```python
from build123d import *

# Parameters (mm, degrees)
BOSS_EXTRUDE1_DEPTH                              = 22.098
BOSS_EXTRUDE2_DEPTH                              = 5.08
FILLET1_R                                        = 2.54
CBORE_FOR_M4_HEX_HEAD_MACHINE_SCREW1_D           = 4.5
CBORE_FOR_M4_HEX_HEAD_MACHINE_SCREW1_CBORE_D     = 10.59
CBORE_FOR_M4_HEX_HEAD_MACHINE_SCREW1_CBORE_DEPTH = 3
M4_CLEARANCE_HOLE1_D                             = 4.8


with BuildPart() as part:
    # Sketch1 → Boss-Extrude1 (new body)
    with BuildSketch(Plane(origin=(0, 0, 0), x_dir=(1, 0, 0), z_dir=(0, 1, 0))):
        with BuildLine():
            Line((-6.35, 4.572), (-6.35, 0))
            Line((-6.35, 0), (6.35, 0))
            Line((6.35, 0), (6.35, 4.572))
            ThreePointArc((6.35, 4.572), (0, 10.922), (-6.35, 4.572))
        make_face()
    extrude(amount=BOSS_EXTRUDE1_DEPTH)

    # Sketch2 → Boss-Extrude2 (add)
    with BuildSketch(Plane(origin=(0, 22.098, 0), x_dir=(1, 0, 0), z_dir=(0, 1, 0))):
        with BuildLine():
            Line((-6.35, 0), (-6.35, -19.05))
            Line((-6.35, -19.05), (6.35, -19.05))
            Line((6.35, -19.05), (6.35, 0))
            Line((6.35, 0), (6.35, 4.572))
            ThreePointArc((6.35, 4.572), (0, 10.922), (-6.35, 4.572))
            Line((-6.35, 4.572), (-6.35, 0))
        make_face()
    extrude(amount=BOSS_EXTRUDE2_DEPTH)

    # Fillet1
    fillet1_edges = [part.edges().sort_by_distance(p)[0] for p in [
        (6.35, 24.638, 19.05),
        (-6.35, 24.638, 19.05),
    ]]
    fillet(fillet1_edges, radius=FILLET1_R)

    # CBORE for M4 Hex Head Machine Screw1 (through all)
    with Locations(Plane(origin=(0, 27.178, 0), x_dir=(1, 0, 0), z_dir=(0, 1, 0))):
        with Locations((0, 4.572)):
            CounterBoreHole(CBORE_FOR_M4_HEX_HEAD_MACHINE_SCREW1_D / 2, CBORE_FOR_M4_HEX_HEAD_MACHINE_SCREW1_CBORE_D / 2, CBORE_FOR_M4_HEX_HEAD_MACHINE_SCREW1_CBORE_DEPTH)

    # M4 Clearance Hole1 (through all)
    with Locations(Plane(origin=(0, 24.178, 0), x_dir=(1, 0, 0), z_dir=(0, 1, 0))):
        with Locations((0, 4.572)):
            Hole(M4_CLEARANCE_HOLE1_D / 2)


solid = part.part
```
Geometry check sheet. Reference: the model listing, model coordinates, mm. A direction names the side the tool comes from. Give positions to 0.01 mm unless a question says otherwise; leave off trailing zeros. Write each loop counter-clockwise with the first axis right and the second up, starting at its lowest first coordinate (ties: lowest second). Pieces come first, ordered by that corner, then holes. Notation, with made-up numbers: (-34.5, -37) -> (-10.5, -37) arc R21 cw to (-10.5, -24) -> close; hole circle Ø10 at (24, 71.5). An arc over 180 degrees is marked (long way). Use one line per item in the form item = value.
Item 1: Depth check by flat-ended pin: pin 1 Ø4 at (x, z) = (0.5, 5) entering from -Y; pin 2 Ø5.5 at (x, z) = (-0.5, -6) entering from +Y; pin 3 Ø1 at (x, y) = (0.5, 9) entering from +Z; pin 4 Ø4 at (x, z) = (0, -4.572) entering from -Y. Enter the tip coordinate at first touch or a pass-through.
Results list:
pin_1 = 22.1
pin_2 = 24.18
pin_3 = 0
pin_4 = through
Item 2: Sectioned sample at B-B on y = 24.75. Enter the section's corners in (x, z) (3 decimals), plus the area to 3 significant figures.
Results list:
outline = (-6.35, -4.572) arc R6.35 ccw to (6.35, -4.572) -> (6.35, 16.51) arc R2.54 ccw to (3.81, 19.05) -> (-3.81, 19.05) arc R2.54 ccw to (-6.35, 16.51) -> close; hole circle Ø10.59 at (0, -4.572)
area = 272 mm2
Item 3: Sectioned sample at D-D on x = -2. Enter the section's corners in (y, z), plus the area to 3 significant figures.
Results list:
outline = (0, -10.6) -> (27.18, -10.6) -> (27.18, -9.47) -> (24.18, -9.47) -> (24.18, -5.9) -> (0, -5.9) -> close; (0, -3.25) -> (24.18, -3.25) -> (24.18, 0.33) -> (27.18, 0.33) -> (27.18, 19.05) -> (22.1, 19.05) -> (22.1, 0) -> (0, 0) -> close
area = 291 mm2
Item 4: Sectioned sample at A-A on x = 0. Enter the section's corners in (y, z).
Results list:
outline = (0, -10.92) -> (27.18, -10.92) -> (27.18, -9.87) -> (24.18, -9.87) -> (24.18, -6.97) -> (0, -6.97) -> close; (0, -2.17) -> (24.18, -2.17) -> (24.18, 0.72) -> (27.18, 0.72) -> (27.18, 19.05) -> (22.1, 19.05) -> (22.1, 0) -> (0, 0) -> close
Item 5: Access from +Z, -Z, +X, -X, +Y, -Y to the whole of each face (thin tool, end or side, straight path). Record for faces 4 (the cylindrical face through (5.586, 24.674, 18.326)), 5 (the cylindrical face through (-0.69, 25.7, -9.82)), 6 (the flat face through (0, 22.098, 9)).
Results list:
face_4 = +Z, +X, +Y, -Y
face_5 = +Y
face_6 = +Z, +X, -X, -Y
Item 6: Scan lines: line 1 (Z direction, x = 0, y = 25.3); line 2 (Z direction, x = -1.75, y = 23.5); line 3 (Y direction, x = -5, z = 9.5). Record each from-to range of solid material in increasing order.
Results list:
line_1 = -10.92 to -9.87, 0.72 to 19.05
line_2 = -10.68 to -6.21, -2.93 to 19.05
line_3 = 22.1 to 27.18
Item 7: Mould release check, pull along Z, two halves, no side actions. Record for faces 1 (the flat face through (6.35, 19, -1)), 2 (the cylindrical face through (-5.586, 24.674, 18.326)), 3 (the flat face through (1, 24.178, -2)): released by +Z, released by -Z, zero draft, split by the parting line, or undercut.
Results list:
face_1 = zero draft
face_2 = released by +Z
face_3 = undercut
Item 8: Sectioned sample at C-C on z = 8. Enter the section's corners in (x, y), plus the area to 3 significant figures.
Results list:
outline = (-6.35, 22.1) -> (6.35, 22.1) -> (6.35, 27.18) -> (-6.35, 27.18) -> close
area = 64.5 mm2
